Here's how the part is built. I have some questions about the finished solid (model axes, mm). Round coordinates to 2 decimals unless told otherwise and drop trailing zeros. Write each loop counter-clockwise with the first axis right and the second up, starting at its lowest first coordinate (ties: lowest second). Pieces come first, ordered by that corner, then holes. Notation, with made-up numbers: (-24.5, 60.25) - (33.5, 60.25) arc R16 ccw to (33.5, 65.25) - close; hole circle Ø11 at (48.5, 46). An arc over 180 degrees is marked (long way). Write item = value, one per line. Start each with the question number.
Item 1: If we section it at C-C (z = 2): Please give me the cut outline in (x, y), and give its area (3 significant figures).
Item 2: If I drill on line 1 along X through (y, z) = (-29.5, 1.65); line 2 along Y through (x, z) = (-27.5, 0.75); line 3 along X through (y, z) = (-36, 1.6), over which ranges is the centre line in solid material (lowest first)? Write a range as [from, to].
Item 3: If we section it at D-D (x = -27.5): Please give me the cut outline in (y, z), and give its area (3 significant figures).
Item 4: Thinking about a two-plate mould opening in Y: for faces 1 (the face through (-11.056, 40.138, 1.232)), 2 (the face through (-1, 1, 2.5)), which applies, pulls with the +Y half, pulls with the -Y half, needs draft (parallel to the pull), parting line crosses it, or undercut?
Item 5: If we section it at B-B (y = -30): Please give me the cut outline in (x, z).
Item 6: If we section it at A-A (x = 12): Please give me the cut outline in (y, z), and give its area (3 significant figures).
```python
from build123d import *

# Parameters (mm, degrees)
CROQUIS1_W              = 140
CROQUIS1_H              = 150
CROQUIS1_R              = 5.95
CROQUIS1_R_2            = 15
CROQUIS1_W_2            = 12.8
CROQUIS1_H_2            = 19
SALIENTE_EXTRUIR1_DEPTH = 2.5


with BuildPart() as part:
    # Croquis1 → Saliente-Extruir1 (new body)
    with BuildSketch(Plane.XY):
        Rectangle(CROQUIS1_W, CROQUIS1_H)
        with Locations((-27.5, -30)):
            Circle(CROQUIS1_R, mode=Mode.SUBTRACT)
        with Locations((0, 30)):
            Circle(CROQUIS1_R_2, mode=Mode.SUBTRACT)
        with Locations((27.5, -30)):
            Rectangle(CROQUIS1_W_2, CROQUIS1_H_2, mode=Mode.SUBTRACT)
    extrude(amount=SALIENTE_EXTRUIR1_DEPTH)


solid = part.part
```
Reply:
q1.outline = (-70, -75) - (70, -75) - (70, 75) - (-70, 75) - close; hole circle Ø11.9 at (-27.5, -30); hole circle Ø30 at (0, 30); hole (21.1, -39.5) - (33.9, -39.5) - (33.9, -20.5) - (21.1, -20.5) - close
q1.area = 19,900 mm2
q2.line_1 = [-70, -33.43], [-21.57, 21.1], [33.9, 70]
q2.line_2 = [-75, -35.95], [-24.05, 75]
q2.line_3 = [-70, 21.1], [33.9, 70]
q3.outline = (-75, 0) - (-35.95, 0) - (-35.95, 2.5) - (-75, 2.5) - close; (-24.05, 0) - (75, 0) - (75, 2.5) - (-24.05, 2.5) - close
q3.area = 345 mm2
q4.face_1 = undercut
q4.face_2 = needs draft
q5.outline = (-70, 0) - (-33.45, 0) - (-33.45, 2.5) - (-70, 2.5) - close; (-21.55, 0) - (21.1, 0) - (21.1, 2.5) - (-21.55, 2.5) - close; (33.9, 0) - (70, 0) - (70, 2.5) - (33.9, 2.5) - close
q6.outline = (-75, 0) - (21, 0) - (21, 2.5) - (-75, 2.5) - close; (39, 0) - (75, 0) - (75, 2.5) - (39, 2.5) - close
q6.area = 330 mm2
